Build history of the part. All positions in model axes, mm. A direction names the side the tool comes from. Give positions to 0.01 mm unless a question says otherwise; leave off trailing zeros. Order: outer loops, then holes, each group sorted by start corner. A loop starts at its lowest first (then second) coordinate and runs counter-clockwise, first axis right, second up. Notation, with made-up numbers: (-5.75, 9.5) - (39.25, 9.5) arc R18 ccw to (39.25, 32.5) - close; hole circle Ø1 at (81, 68.5). An arc over 180 degrees is marked (long way). Write each question's results on one line, items separated by ' | '. Start each with the question number.
from build123d import *

# Parameters (mm, degrees)
BOSS_EXTRUDE1_DEPTH = 25.4
SKETCH4_R           = 6.35
BOSS_EXTRUDE2_DEPTH = 12.7
BOSS_EXTRUDE3_START = 12.7
SKETCH2_R           = 6.35
BOSS_EXTRUDE3_DEPTH = 12.7


with BuildPart() as part:
    # Sketch1 → Boss-Extrude1 (new body)
    with BuildSketch(Plane.XY):
        Polygon((-77.172248804, 33.927432217), (49.827751196, 33.927432217), (49.827751196, 18.687432217), (57.727272727, 18.687432217), (57.727272727, -32.112567783), (50.435406699, -32.112567783), (50.435406699, -47.352567783), (-75.551834131, -47.352567783), (-75.551834131, -27.040669856), (-84.261562998, -27.040669856), (-84.261562998, 20.35645933), (-77.172248804, 20.35645933), align=None)
    extrude(amount=BOSS_EXTRUDE1_DEPTH)

    # Sketch4 → Boss-Extrude2 (add)
    with BuildSketch(Plane(origin=(0, 33.927432217, 0), x_dir=(1, 0, 0), z_dir=(0, 1, 0))):
        with Locations(Location((-50.151834131, -14.306606111, 0), (0, 0, 270))):
            Circle(SKETCH4_R)
        with Locations(Location((25.035406699, -13.388545476, 0), (0, 0, 270))):
            Circle(SKETCH4_R)
    extrude(amount=BOSS_EXTRUDE2_DEPTH)

    # Sketch2 → Boss-Extrude3 (add)
    with BuildSketch(Plane.XZ.offset(47.352567783).offset(BOSS_EXTRUDE3_START)):
        with Locations(Location((-50.151834131, 14.306606111, 0), (0, 0, 90))):
            Circle(SKETCH2_R)
        with Locations(Location((25.035406699, 13.388545476, 0), (0, 0, 90))):
            Circle(SKETCH2_R)
    extrude(amount=-BOSS_EXTRUDE3_DEPTH)


solid = part.part
Item 1: Flat gauge pins, fed straight in: pin 1 Ø10 at (y, z) = (-33, 8.5) entering from -X; pin 2 Ø4.5 at (x, z) = (-81.5, 9.5) entering from -Y; pin 3 Ø11 at (y, z) = (24.5, 13.5) entering from -X; pin 4 Ø1 at (x, z) = (-38, 2.5) entering from +Y. Where does each tip first touch, or does it go through?
Item 2: Cut at A-A, the plane z = 17. List the corners of the cut face in (x, y), then the cut area to 3 significant figures.
Item 3: Cut at D-D, the plane x = -46. List the corners of the cut face in (y, z).
Item 4: Cut at B-B, the plane x = -25.5. List the corners of the cut face in (y, z).
Item 5: Probe line 1 along Y through (x, z) = (-55, 7.5); line 2 along Y through (x, z) = (-76, 6.75); line 3 along X through (y, z) = (-52, 18.75). List the from-to ranges inside material, lowest first. Write a range as from..to.
Item 6: Which spindle directions (+Z, -Z, +X, -X, +Y, -Y) get a long thin tool onto all of the face, cutting with end or side? Do faces 1 (the flat face through (-80, -27.041, 13)), 2 (the cylindrical face through (-43.856, 40.189, 13.48)), 3 (the cylindrical face through (-52.059, -53.791, 20.363)), 4 (the flat face through (49.828, 26, 13)), 5 (the flat face through (-81, 20.356, 13)). Say none if no direction does.
Item 7: Cut at C-C, the plane y = 32. List the corners of the cut face in (x, z), then the cut area to 3 significant figures.
Values found:
1) pin 1: stops at x = -75.55 | pin 2: stops at y = -27.04 | pin 3: stops at x = -84.26 | pin 4: stops at y = 33.93
2) outline: (-84.26, -27.04) - (-75.55, -27.04) - (-75.55, -47.35) - (-55.9, -47.35) - (-55.9, -60.05) - (-44.4, -60.05) - (-44.4, -47.35) - (19.81, -47.35) - (19.81, -60.05) - (30.26, -60.05) - (30.26, -47.35) - (50.44, -47.35) - (50.44, -32.11) - (57.73, -32.11) - (57.73, 18.69) - (49.83, 18.69) - (49.83, 33.93) - (30.26, 33.93) - (30.26, 46.63) - (19.81, 46.63) - (19.81, 33.93) - (-44.4, 33.93) - (-44.4, 46.63) - (-55.9, 46.63) - (-55.9, 33.93) - (-77.17, 33.93) - (-77.17, 20.36) - (-84.26, 20.36) - close | area: 11,600 mm2
3) outline: (-60.05, 9.5) - (-47.35, 9.5) - (-47.35, 0) - (33.93, 0) - (33.93, 9.5) - (46.63, 9.5) - (46.63, 19.11) - (33.93, 19.11) - (33.93, 25.4) - (-47.35, 25.4) - (-47.35, 19.11) - (-60.05, 19.11) - close
4) outline: (-47.35, 0) - (33.93, 0) - (33.93, 25.4) - (-47.35, 25.4) - close
5) line 1: y = -47.35..33.93 | line 2: y = -27.04..33.93 | line 3: x = -54.69..-45.62, 21.63..28.44
6) face 1: +Z, -Z, -X, -Y | face 2: +Y | face 3: -Y | face 4: +Z, -Z, +X, +Y | face 5: +Z, -Z, -X, +Y
7) outline: (-77.17, 0) - (49.83, 0) - (49.83, 25.4) - (-77.17, 25.4) - close | area: 3,230 mm2
